CAD build for the part. Positions are in the model's coordinates, mm. Face numbers are marked on the shaded views. A direction names the side the tool comes from. Coordinates: 2 decimals unless noted, no trailing zeros. Loops run counter-clockwise (first coordinate to the right, second up) from the corner with the lowest first, then second, coordinate; pieces in that order, holes last. Notation, with made-up numbers: (39.5, 56.5) - (54.5, 56.5) arc R21 cw to (54.5, 82.5) - close; hole circle Ø7 at (77.5, 12.25). An arc over 180 degrees is marked (long way). Put each result on its own line as item: value.
```python
from build123d import *

# Parameters (mm, degrees)
ESQUISSE1_R             = 1
BOSS_EXTRU_1_DEPTH      = 10
ESQUISSE2_R             = 2
ENL_V_MAT_EXTRU_1_DEPTH = 8
CHANFREIN1_SIZE         = 2
CHANFREIN2_SIZE         = 0.25


with BuildPart() as part:
    # Esquisse1 → Boss.-Extru.1 (new body)
    with BuildSketch(Plane.XY):
        with BuildLine():
            Line((-10, -3), (10, -3))
            Line((10, -3), (10, -2))
            Line((10, -2), (3.872983346, -2))
            ThreePointArc((3.872983346, -2), (3.082413931, -1.612372436), (2.90473751, -0.75))
            ThreePointArc((2.90473751, -0.75), (0, 3), (-2.90473751, -0.75))
            ThreePointArc((-2.90473751, -0.75), (-3.082413931, -1.612372436), (-3.872983346, -2))
            Line((-3.872983346, -2), (-10, -2))
            Line((-10, -2), (-10, -3))
        make_face()
        Circle(ESQUISSE1_R, mode=Mode.SUBTRACT)
    extrude(amount=BOSS_EXTRU_1_DEPTH)

    # Esquisse2 → Enlèv. mat.-Extru.1 (cut)
    with BuildSketch(Plane.XY.offset(10)):
        Circle(ESQUISSE2_R)
    extrude(amount=-ENL_V_MAT_EXTRU_1_DEPTH, mode=Mode.SUBTRACT)

    # Chanfrein1
    chanfrein1_edges = [part.edges().sort_by_distance(p)[0] for p in [
        (-10, -2.5, 10),
        (10, -2.5, 10),
        (10, -2.5, 0),
        (-10, -2.5, 0),
    ]]
    chamfer(chanfrein1_edges, length=CHANFREIN1_SIZE)

    # Chanfrein2
    chanfrein2_edges = [part.edges().sort_by_distance(p)[0] for p in [
        (-5.936491673, -2, 0),
        (-3.082413931, -1.612372436, 0),
        (-1, 0, 0),
        (3.082413931, -1.612372436, 10),
        (0, 3, 10),
        (-2, 0, 10),
        (0, -3, 10),
        (5.936491673, -2, 10),
        (0, -3, 0),
        (10, -3, 5),
        (-10, -3, 5),
        (9, -3, 9),
        (9, -3, 1),
        (-9, -3, 1),
        (-9, -3, 9),
        (-10, -2, 5),
        (-3.082413931, -1.612372436, 10),
        (-9, -2, 1),
        (-9, -2, 9),
        (5.936491673, -2, 0),
        (10, -2, 5),
        (9, -2, 9),
        (9, -2, 1),
        (-5.936491673, -2, 10),
        (0, 3, 0),
        (3.082413931, -1.612372436, 0),
    ]]
    chamfer(chanfrein2_edges, length=CHANFREIN2_SIZE)


solid = part.part
```
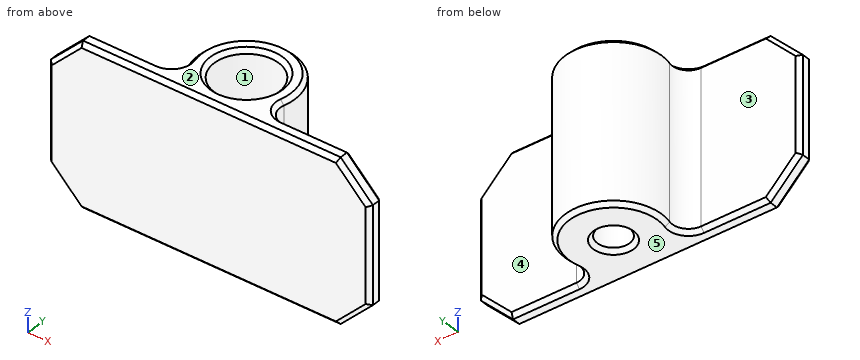
Q1. Pin check, flat tips, straight feed: pin 1 Ø3 at (x, z) = (7.5, 4.5) entering from +Y; pin 2 Ø1.8 at (x, y) = (0, 0) entering from +Z. Stop position of each tip, or through.
Determined:
pin 1: y = -2
pin 2: through
Q2. Tool access for the marked faces 4 and 5: list every direction of +Z, -Z, +X, -X, +Y, -Y with a clear straight run to the whole face (end or side of a thin tool).
Determined:
face 4: +Z, -Z, +X, +Y
face 5: -Z, +X, -X, +Y, -Y
Q3. Mould opens along Y. For the marked faces 1, 2 and 3 say: +Y half, -Y half, draft (parallel to the pull), parting line (faces both ways), or undercut.
Determined:
face 1: undercut
face 2: draft
face 3: +Y half
Q4. Slice it at A-A, the plane x = 0. Give the cut face in (y, z).
Determined:
outline: (-3, 0.25) - (-2.75, 0) - (-1.25, 0) - (-1, 0.25) - (-1, 2) - (-2, 2) - (-2, 9.75) - (-2.25, 10) - (-2.75, 10) - (-3, 9.75) - close; (1, 0.25) - (1.25, 0) - (2.75, 0) - (3, 0.25) - (3, 9.75) - (2.75, 10) - (2.25, 10) - (2, 9.75) - (2, 2) - (1, 2) - close
Q5. Wall check: L1, parallel to X at y = 0, z = 0.85; L2, parallel to Y at x = 6.5, z = 6.25; L3, parallel to X at y = 1, z = 6. Give the ranges that are in metal, low to high. Write a range as from..to.
Determined:
L1: -3..-1, 1..3
L2: -3..-2
L3: -2.83..-1.73, 1.73..2.83
Q6. Slice it at C-C, the plane z = 3. Give the cut face in (x, y).
Determined:
outline: (-10, -2.75) - (-9.75, -3) - (9.75, -3) - (10, -2.75) - (10, -2.25) - (9.75, -2) - (3.87, -2) arc R1 cw to (2.9, -0.75) arc R3 ccw (long way) to (-2.9, -0.75) arc R1 cw to (-3.87, -2) - (-9.75, -2) - (-10, -2.25) - close; hole circle Ø4 at (0, 0)
Q7. Slice it at D-D, the plane y = -2.5. Give the cut face in (x, z), then the cut area to 3 significant figures.
Determined:
outline: (-10, 2) - (-8, 0) - (8, 0) - (10, 2) - (10, 8) - (8, 10) - (-8, 10) - (-10, 8) - close
area: 192 mm2
